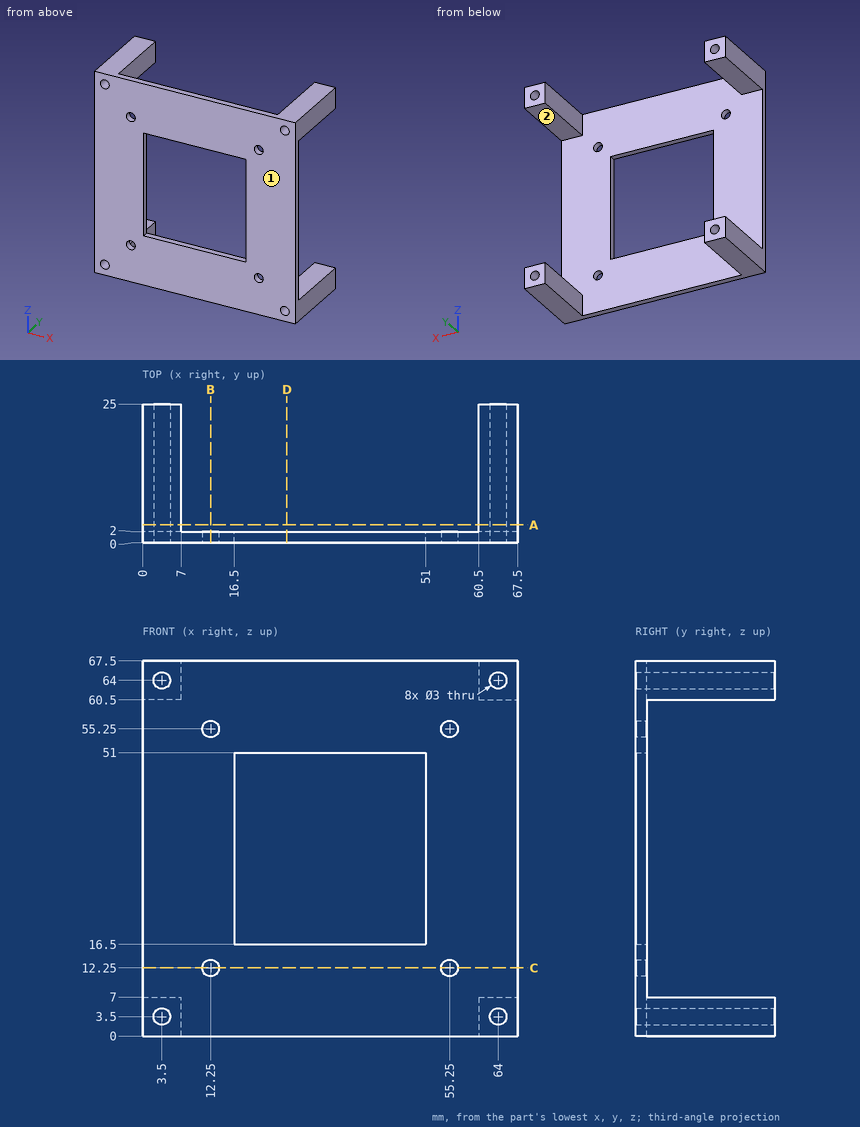
Could you check a few things on this drawing? It's one solid part, dimensions in mm from its lowest x, y, z. A direction names the side the tool comes from. Coordinates: 2 decimals unless noted, no trailing zeros. Order: outer loops, then holes, each group sorted by start corner. A loop starts at its lowest first (then second) coordinate and runs counter-clockwise, first axis right, second up. Notation, with made-up numbers: M -21.75,-4.75 L 13.25,-4.75 A18 cw 13.25,14.25 Z; hole C 27.25,-23.75 d1. An arc over 180 degrees is marked long. Use one line per item in the form item = value. Start each with the question number.
1. Suppose I cut it at B-B on x = 12.25. Write out the boundary of the cut face in (y, z).
2. On a 3-axis mill with a long thin cutter (end or side, diameter ignored), from which of +Z, -Z, +X, -X, +Y, -Y can I reach the whole of each face in a straight line? I mean the marked faces 1 and 2. Say none if no direction works.
3. Suppose I cut it at C-C on z = 12.25. Write out the boundary of the cut face in (x, y), then the cut area to 3 significant figures.
4. For pin 1 (20 mm diameter, centred on x = 43, z = 35, fed in from +Y); pin 2 (7.5 mm diameter, centred on x = 64.5, y = 12.5, fed in from -Z), each with a flat end and sliding along its axis, tell me the tip position at first contact or that it passes through.
5. Please list where these lines run through material, in increasing order: line 1 (X direction, y = 1, z = 55.25); line 2 (X direction, y = 7.5, z = 64); line 3 (Z direction, x = 6.5, y = 12).
6. Suppose I cut it at A-A on y = 3.25. Write out the boundary of the cut face in (x, z).
7. Suppose I cut it at D-D on x = 26. Write out the boundary of the cut face in (y, z).
Geometry says:
q1.outline = M 0,0 L 2,0 L 2,10.75 L 0,10.75 Z; M 0,13.75 L 2,13.75 L 2,53.75 L 0,53.75 Z; M 0,56.75 L 2,56.75 L 2,67.5 L 0,67.5 Z
q2.face_1 = +Z, -Z, +X, -X, -Y
q2.face_2 = +X, -X, +Y
q3.outline = M 0,0 L 10.75,0 L 10.75,2 L 0,2 Z; M 13.75,0 L 53.75,0 L 53.75,2 L 13.75,2 Z; M 56.75,0 L 67.5,0 L 67.5,2 L 56.75,2 Z
q3.area = 123 mm^2
q4.pin_1 = 2
q4.pin_2 = 0
q5.line_1 = 0 to 10.75, 13.75 to 53.75, 56.75 to 67.5
q5.line_2 = 0 to 2, 5 to 7, 60.5 to 62.5, 65.5 to 67.5
q5.line_3 = 0 to 7, 60.5 to 67.5
q6.outline = M 0,0 L 7,0 L 7,7 L 0,7 Z; M 0,60.5 L 7,60.5 L 7,67.5 L 0,67.5 Z; M 60.5,0 L 67.5,0 L 67.5,7 L 60.5,7 Z; M 60.5,60.5 L 67.5,60.5 L 67.5,67.5 L 60.5,67.5 Z; hole C 3.5,3.5 d3; hole C 3.5,64 d3; hole C 64,3.5 d3; hole C 64,64 d3
q7.outline = M 0,0 L 2,0 L 2,16.5 L 0,16.5 Z; M 0,51 L 2,51 L 2,67.5 L 0,67.5 Z
